```python
from build123d import *

# Parameters (mm, degrees)
SKETCH5_R            = 2.794
BOSS_EXTRUDE21_DEPTH = 6.35
SKETCH6_R            = 2.794
CUT_EXTRUDE3_DEPTH   = 6.35


with BuildPart() as part:
    # Sketch5 → Boss-Extrude21 (new body)
    # profile 1 of 3: a face of its own
    with BuildSketch(Plane(origin=(0, 0, 0), x_dir=(1, 0, 0), z_dir=(0, 1, 0))):
        with BuildLine():
            Line((101.6, 12.7), (18.137479686, 12.7))
            Line((18.137479686, 12.7), (11.934096284, -4.34365582))
            ThreePointArc((11.934096284, -4.34365582), (7.284420742, -10.403230962), (0, -12.7))
            Line((0, -12.7), (101.6, -12.7))
            ThreePointArc((101.6, -12.7), (114.3, 0), (101.6, 12.7))
        make_face()
    # profile 2 of 3: a face of its own
    with BuildSketch(Plane(origin=(0, 0, 0), x_dir=(1, 0, 0), z_dir=(0, 1, 0))):
        with BuildLine():
            ThreePointArc((-11.934096284, 4.34365582), (-7.284420742, 10.403230962), (0, 12.7))
            Line((0, 12.7), (18.137479686, 12.7))
            Line((18.137479686, 12.7), (46.683342846, 91.129114452))
            ThreePointArc((46.683342846, 91.129114452), (39.092902382, 107.406866556), (22.815150278, 99.816426092))
            Line((22.815150278, 99.816426092), (-11.934096284, 4.34365582))
        make_face()
    # profile 3 of 3: a face of its own
    with BuildSketch(Plane(origin=(0, 0, 0), x_dir=(1, 0, 0), z_dir=(0, 1, 0))):
        with BuildLine():
            Line((18.137479686, 12.7), (0, 12.7))
            ThreePointArc((0, 12.7), (-7.284420742, 10.403230962), (-11.934096284, 4.34365582))
            ThreePointArc((-11.934096284, 4.34365582), (-10.403230962, -7.284420742), (0, -12.7))
            ThreePointArc((0, -12.7), (7.284420742, -10.403230962), (11.934096284, -4.34365582))
            Line((11.934096284, -4.34365582), (18.137479686, 12.7))
        make_face()
        with Locations(Location((0, 0, 0), (0, 0, 270))):
            Circle(SKETCH5_R, mode=Mode.SUBTRACT)
    extrude(amount=BOSS_EXTRUDE21_DEPTH)

    # Sketch6 → Cut-Extrude3 (cut)
    with BuildSketch(Plane(origin=(0, 0, 0), x_dir=(-1, 0, 0), z_dir=(0, -1, 0))):
        with Locations(Location((-50.8, 0, 0), (0, 0, 90))):
            Circle(SKETCH6_R)
        with Locations(Location((-18.489687901, 50.8, 0), (0, 0, 90))):
            Circle(SKETCH6_R)
    extrude(amount=-CUT_EXTRUDE3_DEPTH, mode=Mode.SUBTRACT)


solid = part.part
```
Work out the finished part from the listing and answer in its coordinate system (mm). A direction names the side the tool comes from. Round coordinates to 2 decimals unless told otherwise and drop trailing zeros. Loops run counter-clockwise (first coordinate to the right, second up) from the corner with the lowest first, then second, coordinate; pieces in that order, holes last. Notation, with made-up numbers: (75.5, -6) -> (119.5, -6) arc R27 cw to (119.5, 17) -> close; hole circle Ø2 at (-18, -26). An arc over 180 degrees is marked (long way). Write each question's results on one line, items separated by ' | '. Start each with the question number.
1. Section A-A (z = 0) is taken. Determine the outline of the cut face in (x, y).
2. A tool of negligible diameter and unlimited length cuts with its end or side. For faces 4 (the face through (32.211, 3.131, -51.366)), 5 (the face through (5.684, 3.131, -52.748)), from which of +Z, -Z, +X, -X, +Y, -Y can it reach the whole face along a straight path? Write none if from no direction.
3. Section C-C (z = -50.8) is taken. Determine the outline of the cut face in (x, y).
4. Given pin 1 Ø1 at (y, z) = (2, -78.5) entering from -X; pin 2 Ø2 at (y, z) = (2.5, -80) entering from +X, each flat-ended and moving along its own axis, determine where each tip first touches the part or whether it passes through.
5. Find the intervals of material crossed by probe 1 along X at (y, z) = (5, 0); probe 2 along Z at (x, y) = (51, 5.75); probe 3 along Z at (x, y) = (55, 5), in increasing order. Write a range as from..to.
6. For a pull along X with two mould halves and no side action, classify faces 1 (the face through (50, 3, 12.7)), 2 (the face through (53.57, 3.13, 0.36)), 3 (the face through (39.35, 3.13, -107.31)) as +X half, -X half, draft (parallel to the pull), parting line (faces both ways), or undercut.
7. Section B-B (x = 50.8) is taken. Determine the outline of the cut face in (y, z), plus the area to 3 significant figures.
8. Section D-D (y = 3.25) is taken. Determine the outline of the cut face in (x, z), plus the area to 3 significant figures.
Evaluation:
1) outline: (-12.7, 0) -> (-2.79, 0) -> (-2.79, 6.35) -> (-12.7, 6.35) -> close; (2.79, 0) -> (48.01, 0) -> (48.01, 6.35) -> (2.79, 6.35) -> close; (53.59, 0) -> (114.3, 0) -> (114.3, 6.35) -> (53.59, 6.35) -> close
2) face 4: +X, +Y, -Y | face 5: -Z, -X, +Y, -Y
3) outline: (4.97, 0) -> (15.7, 0) -> (15.7, 6.35) -> (4.97, 6.35) -> close; (21.28, 0) -> (32, 0) -> (32, 6.35) -> (21.28, 6.35) -> close
4) pin 1: stops at x = 14.87 | pin 2: stops at x = 43
5) probe 1: x = -12.7..-2.79, 2.79..48.01, 53.59..114.3 | probe 2: z = -12.7..-2.79, 2.79..12.7 | probe 3: z = -12.7..12.7
6) face 1: draft | face 2: undercut | face 3: parting line
7) outline: (0, -12.7) -> (6.35, -12.7) -> (6.35, -2.79) -> (0, -2.79) -> close; (0, 2.79) -> (6.35, 2.79) -> (6.35, 12.7) -> (0, 12.7) -> close | area: 126 mm2
8) outline: (-11.93, -4.34) -> (22.82, -99.82) arc R12.7 ccw to (46.68, -91.13) -> (18.14, -12.7) -> (101.6, -12.7) arc R12.7 ccw to (101.6, 12.7) -> (0, 12.7) arc R12.7 ccw to start; hole circle Ø5.59 at (0, 0); hole circle Ø5.59 at (18.49, -50.8); hole circle Ø5.59 at (50.8, 0) | area: 5,520 mm2
